Geometry check sheet. Reference: the model listing, model coordinates, mm. A direction names the side the tool comes from. Coordinates: 2 decimals unless noted, no trailing zeros. Loops run counter-clockwise (first coordinate to the right, second up) from the corner with the lowest first, then second, coordinate; pieces in that order, holes last.
from build123d import *

# Parameters (mm, degrees)
F0_W     = 25
F0_H     = 31
F1_DEPTH = 17
F2_T     = -2
F3_W     = 8
F3_H     = 2
F3_W_2   = 12
F4_DEPTH = 12


with BuildPart() as f1:
    # F0 (on Top) → F1 (new body)
    with BuildSketch(Plane.XY):
        with Locations((-23.056051, 5.904353)):
            Rectangle(F0_W, F0_H)
    extrude(amount=F1_DEPTH)

    # F2
    f2_openings = [f1.faces().sort_by_distance(p)[0] for p in [
        (-23.056051, 5.904353, 17),
    ]]
    offset(amount=F2_T, openings=f2_openings)

    # F3 (on face) → F4 (cut)
    with BuildSketch(Plane.XY.offset(17)):
        with Locations((-24.556051, -8.595647)):
            Rectangle(F3_W, F3_H)
        with Locations((-27.556051, 20.404353)):
            Rectangle(F3_W_2, F3_H)
    extrude(amount=-F4_DEPTH, mode=Mode.SUBTRACT)


solid = f1.part
(1) Sectioned sample at D-D on y = 0.5. Record the cut outline in (x, z), and give its area (3 significant figures).
Findings:
outline: (-35.56, 0) - (-10.56, 0) - (-10.56, 17) - (-12.56, 17) - (-12.56, 2) - (-33.56, 2) - (-33.56, 17) - (-35.56, 17) - close
area: 110 mm2
(2) Gauge pin test, flat ends, axial feed: pin 1 Ø2 at (x, y) = (-26.5, -8.5) entering from +Z; pin 2 Ø8 at (x, z) = (-27.5, 10) entering from +Y; pin 3 Ø4 at (x, y) = (-22.5, 4) entering from +Z. Record the tip position at first contact, or that the pin passes through.
Findings:
pin 1: stops at z = 5
pin 2: stops at y = -7.6
pin 3: stops at z = 2
(3) Draft check along Y on faces 1 (the flat face through (-20, 21.404, 6)), 2 (the flat face through (-23, 6, 2)), 3 (the flat face through (-25, -9, 5)). Enter one of: +Y half, -Y half, draft (parallel to the pull), parting line (faces both ways), or undercut.
Findings:
face 1: +Y half
face 2: undercut
face 3: draft
(4) Scan lines: L1, parallel to Y at x = -12.75, z = 16; L2, parallel to X at y = 15.5, z = 10; L3, parallel to X at y = -8, z = 14.75. Record each from-to range of solid material in increasing order.
Findings:
L1: y = -9.6 to -7.6, 19.4 to 21.4
L2: x = -35.56 to -33.56, -12.56 to -10.56
L3: x = -35.56 to -28.56, -20.56 to -10.56
(5) Access from +Z, -Z, +X, -X, +Y, -Y to the whole of each face (thin tool, end or side, straight path). Record for faces 4 (the flat face through (-12.556, 6, 9)), 5 (the flat face through (-21.556, 20, 11)), 6 (the flat face through (-28, 20, 5)).
Findings:
face 4: +Z
face 5: +Z, +Y, -Y
face 6: +Z, +Y
(6) Sectioned sample at B-B on z = 4. Record the cut outline in (x, y), and give its area (3 significant figures).
Findings:
outline: (-35.56, -9.6) - (-10.56, -9.6) - (-10.56, 21.4) - (-35.56, 21.4) - close; hole (-33.56, -7.6) - (-12.56, -7.6) - (-12.56, 19.4) - (-33.56, 19.4) - close
area: 208 mm2
(7) Sectioned sample at C-C on x = -24.75. Record the cut outline in (y, z), and give its area (3 significant figures).
Findings:
outline: (-9.6, 0) - (21.4, 0) - (21.4, 5) - (19.4, 5) - (19.4, 2) - (-7.6, 2) - (-7.6, 5) - (-9.6, 5) - close
area: 74.0 mm2
(8) Sectioned sample at A-A on z = 13.75. Record the cut outline in (x, y).
Findings:
outline: (-35.56, -9.6) - (-28.56, -9.6) - (-28.56, -7.6) - (-33.56, -7.6) - (-33.56, 21.4) - (-35.56, 21.4) - close; (-21.56, 19.4) - (-12.56, 19.4) - (-12.56, -7.6) - (-20.56, -7.6) - (-20.56, -9.6) - (-10.56, -9.6) - (-10.56, 21.4) - (-21.56, 21.4) - close
